The listing builds one solid part. Answer for the finished solid, in the listing's coordinates (mm). A direction names the side the tool comes from. Coordinates: 2 decimals unless noted, no trailing zeros. Order: outer loops, then holes, each group sorted by start corner. A loop starts at its lowest first (then second) coordinate and runs counter-clockwise, first axis right, second up. Notation, with made-up numbers: (45, 53) -> (81, 53) arc R23 ccw to (81, 66) -> close; hole circle Ø7 at (41, -17.5). An arc over 180 degrees is marked (long way). Answer in a Markdown table with one row per item. Add a question column.
```python
from build123d import *

# Parameters (mm, degrees)
SKETCH_W             = 185.32
SKETCH_H             = 240.5
PAD_DEPTH            = 30
SKETCH003_W          = 145.32
SKETCH003_H          = 200.5
POCKET_DEPTH         = 23.6
SKETCH004_W          = 80.32
SKETCH004_H          = 135.5
POCKET001_DEPTH      = 6.4
POCKET002_DEPTH      = 3
SKETCH006_W          = 14
SKETCH006_H          = 3
POCKET003_DEPTH      = 30
POCKET004_DEPTH      = 1.5
SKETCH008_W          = 12
SKETCH008_H          = 2.4244
POCKET005_DEPTH      = 30
SKETCH009_W          = 87.32
SKETCH009_H          = 142.5
PAD001_DEPTH         = 4
SKETCH010_W          = 76.32
SKETCH010_H          = 131.5
POCKET006_DEPTH      = 0.001
POCKET006_DEPTH_BACK = -30.001
CHAMFER_SIZE         = 10
CHAMFER001_SIZE      = 5
CHAMFER002_SIZE      = 2


with BuildPart() as part:
    # Sketch → Pad (new body)
    with BuildSketch(Plane.XY):
        Rectangle(SKETCH_W, SKETCH_H)
    extrude(amount=PAD_DEPTH)

    # Sketch003 → Pocket (cut)
    with BuildSketch(Plane.XY.offset(30)):
        Rectangle(SKETCH003_W, SKETCH003_H)
    extrude(amount=-POCKET_DEPTH, mode=Mode.SUBTRACT)

    # Sketch004 → Pocket001 (cut)
    with BuildSketch(Plane.XY.offset(6.4)):
        Rectangle(SKETCH004_W, SKETCH004_H)
    extrude(amount=-POCKET001_DEPTH, mode=Mode.SUBTRACT)

    # Sketch005 → Pocket002 (cut)
    with BuildSketch(Plane.XY):
        with BuildLine():
            ThreePointArc((-85.97, 0), (-82.985, -2.985), (-80, 0))
            Line((-80, 0), (-80, 18.025988))
            ThreePointArc((-80, 18.025988), (-82.985, 27.495), (-85.97, 18.025988))
            Line((-85.97, 18.025988), (-85.97, 0))
        make_face()
    extrude(amount=POCKET002_DEPTH, mode=Mode.SUBTRACT)

    # Sketch006 → Pocket003 (cut, symmetric)
    with BuildSketch(Plane.XZ):
        with Locations((-83, 4.48)):
            Rectangle(SKETCH006_W, SKETCH006_H)
    extrude(amount=POCKET003_DEPTH, both=True, mode=Mode.SUBTRACT)

    # Sketch007 → Pocket004 (cut, symmetric)
    with BuildSketch(Plane.XY):
        with BuildLine():
            ThreePointArc((0, 110.985), (-2.985, 108), (0, 105.015))
            Line((0, 105.015), (18.705988, 105.015))
            ThreePointArc((18.705988, 105.015), (28.175, 108), (18.705988, 110.985))
            Line((18.705988, 110.985), (0, 110.985))
        make_face()
    extrude(amount=POCKET004_DEPTH, both=True, mode=Mode.SUBTRACT)

    # Sketch008 → Pocket005 (cut, symmetric)
    with BuildSketch(Plane.YZ):
        with Locations((108, 2.7105)):
            Rectangle(SKETCH008_W, SKETCH008_H)
    extrude(amount=POCKET005_DEPTH, both=True, mode=Mode.SUBTRACT)

    # Sketch009 → Pad001 (join)
    with BuildSketch(Plane.XY.offset(6.4)):
        Rectangle(SKETCH009_W, SKETCH009_H)
    extrude(amount=PAD001_DEPTH)

    # Sketch010 → Pocket006 (cut, two sides)
    with BuildSketch(Plane.XY) as pocket006_sk:
        Rectangle(SKETCH010_W, SKETCH010_H)
    extrude(amount=-POCKET006_DEPTH, mode=Mode.SUBTRACT)
    extrude(pocket006_sk.sketch, amount=-POCKET006_DEPTH_BACK, mode=Mode.SUBTRACT)

    # Chamfer
    chamfer_edges = [part.edges().sort_by_distance(p)[0] for p in [
        (-72.66, 0, 30),
        (0, 100.25, 30),
        (72.66, 0, 30),
        (0, -100.25, 30),
    ]]
    chamfer(chamfer_edges, length=CHAMFER_SIZE)

    # Chamfer001
    chamfer001_edges = [part.edges().sort_by_distance(p)[0] for p in [
        (0, 120.25, 30),
        (-92.66, 0, 30),
        (0, -120.25, 30),
        (92.66, 0, 30),
    ]]
    chamfer(chamfer001_edges, length=CHAMFER001_SIZE)

    # Chamfer002
    chamfer002_edges = [part.edges().sort_by_distance(p)[0] for p in [
        (-43.66, 0, 10.4),
        (0, -71.25, 10.4),
        (43.66, 0, 10.4),
        (0, 71.25, 10.4),
    ]]
    chamfer(chamfer002_edges, length=CHAMFER002_SIZE)


solid = part.part
```
Q1. For faces 4 (the face through (0, 108, 3.923)), 5 (the face through (-1, 120.25, 12)), 6 (the face through (-40.16, -1, 3)), 7 (the face through (-77.73, -1.54, 25.07)), 8 (the face through (-92.66, -2, 12)), determine the directions among +Z, -Z, +X, -X, +Y, -Y from which every point of the face is accessible in a straight line to the end or side of a thin tool.
Q2. Determine the mould class of faces 1 (the face through (-1.3, -117.79, 27.46)), 2 (the face through (-90.2, -1.68, 27.46)), 3 (the face through (-83, 0, 5.98)) for opening direction Y: +Y half, -Y half, draft (parallel to the pull), parting line (faces both ways), or undercut.
Q3. A cutting plane is placed at C-C (y = 36.5). Determine the outline of the cut face in (x, z), then the cut area to 3 significant figures.
Q4. A cutting plane is placed at B-B (z = 13). Determine the outline of the cut face in (x, y).
Q5. A cutting plane is placed at A-A (x = -23.5). State how many separate pieces and enclosed holes the cut face has, then the cut area to 3 significant figures.
Q6. Straight lines are drawn through the part: line 1 (Y direction, x = 22.97, z = 0.4) (3 decimals); line 2 (X direction, y = 22.29, z = 1); line 3 (X direction, y = -51.5, z = 6). For each, find the intervals that lie inside material, in ascending order.
Q7. Given pin 1 (8 mm diameter, centred on x = 47.5, y = 57.5, fed in from -Z); pin 2 (1 mm diameter, centred on x = 62, y = 84, fed in from +Z), each flat-ended and moving along its own axis, determine where each tip first touches the part or whether it passes through.
Returned:
| question | item | result |
|---|---|---|
| 1 | face 4 | none |
| 1 | face 5 | +Z, -Z, +X, -X, +Y |
| 1 | face 6 | -Z |
| 1 | face 7 | +Z |
| 1 | face 8 | +Z, -Z, -X, +Y, -Y |
| 2 | face 1 | -Y half |
| 2 | face 2 | draft |
| 2 | face 3 | undercut |
| 3 | outline | (-92.66, 0) -> (-40.16, 0) -> (-40.16, 6.4) -> (-38.16, 6.4) -> (-38.16, 10.4) -> (-41.66, 10.4) -> (-43.66, 8.4) -> (-43.66, 6.4) -> (-72.66, 6.4) -> (-72.66, 20) -> (-82.66, 30) -> (-87.66, 30) -> (-92.66, 25) -> close; (38.16, 6.4) -> (40.16, 6.4) -> (40.16, 0) -> (92.66, 0) -> (92.66, 25) -> (87.66, 30) -> (82.66, 30) -> (72.66, 20) -> (72.66, 6.4) -> (43.66, 6.4) -> (43.66, 8.4) -> (41.66, 10.4) -> (38.16, 10.4) -> close |
| 3 | area | 1,530 mm² |
| 4 | outline | (-92.66, -120.25) -> (92.66, -120.25) -> (92.66, 120.25) -> (-92.66, 120.25) -> close; hole (-72.66, -100.25) -> (72.66, -100.25) -> (72.66, 100.25) -> (-72.66, 100.25) -> close |
| 5 | separate pieces | 2 |
| 5 | enclosed holes | 1 |
| 5 | area | 1,500 mm² |
| 6 | line 1 | y = -120.25 to -67.75, 67.75 to 102.795, 113.205 to 120.25 |
| 6 | line 2 | x = -92.66 to -88.19, -77.78 to -40.16, 40.16 to 92.66 |
| 6 | line 3 | x = -92.66 to -40.16, 40.16 to 92.66 |
| 7 | pin 1 | stops at z = 0 |
| 7 | pin 2 | stops at z = 6.4 |
